```python
from build123d import *

# Parameters (mm, degrees)
SKETCH1_R           = 5.75
BOSS_EXTRUDE1_DEPTH = 10
SKETCH2_W           = 16
SKETCH2_H           = 2.5
BOSS_EXTRUDE2_DEPTH = 2


with BuildPart() as part:
    # Sketch1 → Boss-Extrude1 (new body)
    with BuildSketch(Plane(origin=(0, 0, 0), x_dir=(1, 0, 0), z_dir=(0, 1, 0))):
        Circle(SKETCH1_R)
    extrude(amount=BOSS_EXTRUDE1_DEPTH)

    # Sketch2 → Boss-Extrude2 (add)
    with BuildSketch(Plane(origin=(0, 0, 0), x_dir=(-1, 0, 0), z_dir=(0, -1, 0))):
        Rectangle(SKETCH2_W, SKETCH2_H)
    extrude(amount=-BOSS_EXTRUDE2_DEPTH)


solid = part.part
```
The model under review builds one solid part; all positions refer to its coordinate system, in mm. A direction names the side the tool comes from. Round coordinates to 2 decimals unless told otherwise and drop trailing zeros. Write each loop counter-clockwise with the first axis right and the second up, starting at its lowest first coordinate (ties: lowest second). Pieces come first, ordered by that corner, then holes.
(1) We need section B-B on y = 1.75. Give the boundary of the cut face in (x, z), and give its area (3 significant figures).
(2) We need section A-A on z = 0. Give the boundary of the cut face in (x, y).
(3) Insertion check: pin 1 (3 mm diameter, centred on y = 5, z = 3.5, fed in from -X); pin 2 (1.5 mm diameter, centred on y = 3, z = -2.5, fed in from -X); pin 3 (0.7 mm diameter, centred on x = 7, z = -0.5, fed in from +Y); pin 4 (5 mm diameter, centred on x = -1.5, y = 8, fed in from -Z). Each pin has a flat end and moves straight along its axis. Give the tip position at first contact, or say it passes through.
(4) We need section D-D on y = 9. Give the boundary of the cut face in (x, z).
(5) Machinability: for faces 1 (the flat face through (8, 1, 0)), 2 (the flat face through (-7, 1, 1.25)), 3 (the flat face through (-7, 1, -1.25)), 4 (the flat face through (7, 1, 1.25)), 5 (the flat face through (7, 1, -1.25)), which of the approach directions +Z, -Z, +X, -X, +Y, -Y give a long, thin tool a straight path to every point of the face, cutting with its end or side? Answer none if there is none.
(6) We need section C-C on x = -6.5. Give the boundary of the cut face in (y, z), and give its area (3 significant figures).
(7) Wall thickness on L1, parallel to X at y = 9.75, z = -1.25; L2, parallel to Z at x = 4.25, y = 5.75: over which ranges is each line inside the solid? List them lowest first.
Findings below:
1. outline: (-8, -1.25) - (-5.61, -1.25) arc R5.75 ccw to (5.61, -1.25) - (8, -1.25) - (8, 1.25) - (5.61, 1.25) arc R5.75 ccw to (-5.61, 1.25) - (-8, 1.25) - close
1. area: 115 mm2
2. outline: (-8, 0) - (8, 0) - (8, 2) - (5.75, 2) - (5.75, 10) - (-5.75, 10) - (-5.75, 2) - (-8, 2) - close
3. pin 1: stops at x = -5.39
3. pin 2: stops at x = -5.48
3. pin 3: stops at y = 2
3. pin 4: stops at z = -5.75
4. outline: circle Ø11.5 at (0, 0)
5. face 1: +Z, -Z, +X, +Y, -Y
5. face 2: +Z, -X, +Y, -Y
5. face 3: -Z, -X, +Y, -Y
5. face 4: +Z, +X, +Y, -Y
5. face 5: -Z, +X, +Y, -Y
6. outline: (0, -1.25) - (2, -1.25) - (2, 1.25) - (0, 1.25) - close
6. area: 5.00 mm2
7. L1: x = -5.61 to 5.61
7. L2: z = -3.87 to 3.87
